```python
from build123d import *

# Parameters (mm, degrees)
BOSS_EXTRUDE1_DEPTH = 3.175
BOSS_EXTRUDE2_DEPTH = 6.35
CAVITY2_START       = -95.885
CAVITY2_OUTLINE_W   = 6.35
CAVITY2_OUTLINE_H   = 6.35
CAVITY2_DEPTH       = 15.875
CAVITY2_START_2     = -64.135
CAVITY2_2_OUTLINE_W = 6.35
CAVITY2_2_OUTLINE_H = 6.35
CAVITY2_2_DEPTH     = 15.875
SKETCH6_R           = 1.3716
CUT_EXTRUDE1_DEPTH  = 175.52022504
SKETCH7_R           = 6.35
CUT_EXTRUDE2_DEPTH  = 175.52022504
SKETCH9_R           = 1.905
CUT_EXTRUDE3_DEPTH  = 175.52022504
SKETCH10_R          = 1.85
CUT_EXTRUDE4_DEPTH  = 175.52022504
CAVITY3_START       = 48.26
CAVITY3_OUTLINE_W   = 6.35
CAVITY3_OUTLINE_H   = 6.35
CAVITY3_DEPTH       = 15.875
CAVITY3_START_2     = 80.01
CAVITY3_2_OUTLINE_W = 6.35
CAVITY3_2_OUTLINE_H = 6.35
CAVITY3_2_DEPTH     = 15.875
CAVITY3_START_3     = -95.885
CAVITY3_3_OUTLINE_W = 6.35
CAVITY3_3_OUTLINE_H = 6.35
CAVITY3_3_DEPTH     = 15.875
CAVITY3_START_4     = -64.135
CAVITY3_4_OUTLINE_W = 6.35
CAVITY3_4_OUTLINE_H = 6.35
CAVITY3_4_DEPTH     = 15.875
CAVITY3_START_5     = -114.3
CAVITY3_5_OUTLINE_W = 6.35
CAVITY3_5_OUTLINE_H = 11.6205
CAVITY3_5_DEPTH     = 2.54
CAVITY3_START_6     = 111.76
CAVITY3_6_OUTLINE_W = 6.35
CAVITY3_6_OUTLINE_H = 11.6205
CAVITY3_6_DEPTH     = 2.54


# Read off the part's stored shape, not the designer's step: Cavity2, Cavity3
with BuildPart() as part:
    # Sketch1 → Boss-Extrude1 (new, symmetric)
    with BuildSketch(Plane(origin=(0, 0, 0), x_dir=(1, 0, 0), z_dir=(0, 1, 0))):
        Polygon((9.874658932, 123.322719821), (-80.219893167, 94.184769753), (-123.322719821, 9.874658932), (-94.184769753, -80.219893167), (-9.874658932, -123.322719821), (80.219893167, -94.184769753), (123.322719821, -9.874658932), (94.184769753, 80.219893167), align=None)
    extrude(amount=BOSS_EXTRUDE1_DEPTH, both=True)

    # Sketch3 → Boss-Extrude2 (add)
    with BuildSketch(Plane(origin=(0, 3.175, 0), x_dir=(1, 0, 0), z_dir=(0, 1, 0))):
        Polygon((95.310120051, 76.74030964), (117.060869008, 83.774833064), (106.89989073, 115.192581558), (57.210976805, 99.122430154), (94.184769753, 80.219893167), align=None)
    extrude(amount=-BOSS_EXTRUDE2_DEPTH)

    # Cavity2 outline → Cavity2 (cut)
    with BuildSketch(Plane(origin=(0, 0, 0), x_dir=(0, 1, 0), z_dir=(0.9514763323416664, 0, -0.3077219345344931)).offset(CAVITY2_START)):
        with Locations((0, 26.416)):
            Rectangle(CAVITY2_OUTLINE_W, CAVITY2_OUTLINE_H)
    extrude(amount=CAVITY2_DEPTH, mode=Mode.SUBTRACT)

    # Cavity2 2 outline → Cavity2 2 (cut)
    with BuildSketch(Plane(origin=(0, 0, 0), x_dir=(0, 1, 0), z_dir=(0.9514763323416664, 0, -0.3077219345344931)).offset(CAVITY2_START_2)):
        with Locations((0, 26.416)):
            Rectangle(CAVITY2_2_OUTLINE_W, CAVITY2_2_OUTLINE_H)
    extrude(amount=CAVITY2_2_DEPTH, mode=Mode.SUBTRACT)

    # Sketch6 → Cut-Extrude1 (cut, through all)
    with BuildSketch(Plane(origin=(0, 3.175, 0), x_dir=(1, 0, 0), z_dir=(0, 1, 0))):
        with Locations(Location((-5.097490915, -79.318746248, 0), (0, 0, 270))):
            Circle(SKETCH6_R)
        with Locations(Location((50.579592916, -61.311929511, 0), (0, 0, 270))):
            Circle(SKETCH6_R)
        with Locations(Location((34.017198322, -10.100999466, 0), (0, 0, 270))):
            Circle(SKETCH6_R)
        with Locations(Location((-21.659885509, -28.107816203, 0), (0, 0, 270))):
            Circle(SKETCH6_R)
    extrude(amount=-CUT_EXTRUDE1_DEPTH, mode=Mode.SUBTRACT)

    # Sketch7 → Cut-Extrude2 (cut, through all)
    with BuildSketch(Plane(origin=(0, 3.175, 0), x_dir=(1, 0, 0), z_dir=(0, 1, 0))):
        with Locations(Location((56.160215938, -31.223340716, 0), (0, 0, 270))):
            Circle(SKETCH7_R)
    extrude(amount=-CUT_EXTRUDE2_DEPTH, mode=Mode.SUBTRACT)

    # Sketch9 → Cut-Extrude3 (cut, through all)
    with BuildSketch(Plane(origin=(0, 3.175, 0), x_dir=(1, 0, 0), z_dir=(0, 1, 0))):
        with Locations(Location((-19.963200574, -76.531714164, 0), (0, 0, 270))):
            Circle(SKETCH9_R)
        with Locations(Location((-41.457577702, -10.07109235, 0), (0, 0, 270))):
            Circle(SKETCH9_R)
        with Locations(Location((60.997920545, -50.347654754, 0), (0, 0, 270))):
            Circle(SKETCH9_R)
        with Locations(Location((39.503543417, 16.11296706, 0), (0, 0, 270))):
            Circle(SKETCH9_R)
    extrude(amount=-CUT_EXTRUDE3_DEPTH, mode=Mode.SUBTRACT)

    # Sketch10 → Cut-Extrude4 (cut, through all)
    with BuildSketch(Plane(origin=(0, 3.175, 0), x_dir=(1, 0, 0), z_dir=(0, 1, 0))):
        with Locations(Location((-1.658619289, 61.997975629, 0), (0, 0, 270))):
            Circle(SKETCH10_R)
        with Locations(Location((-34.960290921, 51.22770792, 0), (0, 0, 270))):
            Circle(SKETCH10_R)
        with Locations(Location((-23.574579343, 16.023083623, 0), (0, 0, 270))):
            Circle(SKETCH10_R)
        with Locations(Location((9.727092289, 26.793351332, 0), (0, 0, 270))):
            Circle(SKETCH10_R)
    extrude(amount=-CUT_EXTRUDE4_DEPTH, mode=Mode.SUBTRACT)

    # Cavity3 outline → Cavity3 (cut)
    with BuildSketch(Plane(origin=(0, 0, 0), x_dir=(0, 1, 0), z_dir=(0.9514763323416664, 0, -0.3077219345344931)).offset(CAVITY3_START)):
        with Locations((0, 26.416)):
            Rectangle(CAVITY3_OUTLINE_W, CAVITY3_OUTLINE_H)
        with Locations((0, -26.416)):
            Rectangle(CAVITY3_OUTLINE_W, CAVITY3_OUTLINE_H)
    extrude(amount=CAVITY3_DEPTH, mode=Mode.SUBTRACT)

    # Cavity3 2 outline → Cavity3 2 (cut)
    with BuildSketch(Plane(origin=(0, 0, 0), x_dir=(0, 1, 0), z_dir=(0.9514763323416664, 0, -0.3077219345344931)).offset(CAVITY3_START_2)):
        with Locations((0, 26.416)):
            Rectangle(CAVITY3_2_OUTLINE_W, CAVITY3_2_OUTLINE_H)
        with Locations((0, -26.416)):
            Rectangle(CAVITY3_2_OUTLINE_W, CAVITY3_2_OUTLINE_H)
    extrude(amount=CAVITY3_2_DEPTH, mode=Mode.SUBTRACT)

    # Cavity3 3 outline → Cavity3 3 (cut)
    with BuildSketch(Plane(origin=(0, 0, 0), x_dir=(0, 1, 0), z_dir=(0.9514763323416664, 0, -0.3077219345344931)).offset(CAVITY3_START_3)):
        with Locations((0, -26.416)):
            Rectangle(CAVITY3_3_OUTLINE_W, CAVITY3_3_OUTLINE_H)
    extrude(amount=CAVITY3_3_DEPTH, mode=Mode.SUBTRACT)

    # Cavity3 4 outline → Cavity3 4 (cut)
    with BuildSketch(Plane(origin=(0, 0, 0), x_dir=(0, 1, 0), z_dir=(0.9514763323416664, 0, -0.3077219345344931)).offset(CAVITY3_START_4)):
        with Locations((0, -26.416)):
            Rectangle(CAVITY3_4_OUTLINE_W, CAVITY3_4_OUTLINE_H)
    extrude(amount=CAVITY3_4_DEPTH, mode=Mode.SUBTRACT)

    # Cavity3 5 outline → Cavity3 5 (cut)
    with BuildSketch(Plane(origin=(0, 0, 0), x_dir=(0, 1, 0), z_dir=(0.9514763323416664, 0, -0.3077219345344931)).offset(CAVITY3_START_5)):
        with Locations((0, 17.43075)):
            Rectangle(CAVITY3_5_OUTLINE_W, CAVITY3_5_OUTLINE_H)
        with Locations((0, -17.43075)):
            Rectangle(CAVITY3_5_OUTLINE_W, CAVITY3_5_OUTLINE_H)
    extrude(amount=CAVITY3_5_DEPTH, mode=Mode.SUBTRACT)

    # Cavity3 6 outline → Cavity3 6 (cut)
    with BuildSketch(Plane(origin=(0, 0, 0), x_dir=(0, 1, 0), z_dir=(0.9514763323416664, 0, -0.3077219345344931)).offset(CAVITY3_START_6)):
        with Locations((0, 17.43075)):
            Rectangle(CAVITY3_6_OUTLINE_W, CAVITY3_6_OUTLINE_H)
        with Locations((0, -17.43075)):
            Rectangle(CAVITY3_6_OUTLINE_W, CAVITY3_6_OUTLINE_H)
    extrude(amount=CAVITY3_6_DEPTH, mode=Mode.SUBTRACT)


solid = part.part
```
Geometry check sheet. Reference: the model listing, model coordinates, mm. A direction names the side the tool comes from. Coordinates: 2 decimals unless noted, no trailing zeros. Order: outer loops, then holes, each group sorted by start corner. A loop starts at its lowest first (then second) coordinate and runs counter-clockwise, first axis right, second up.
Q1. Sectioned sample at C-C on z = -88. Record the cut outline in (x, y) (3 decimals), and give its area (3 significant figures).
Reply:
outline: (-83.382, -3.175) - (115.694, -3.175) - (115.694, 3.175) - (-83.382, 3.175) - close
area: 1,260 mm2
Q2. Thickness scan on probe 1 along Z at (x, y) = (-41, 2.75); probe 2 along X at (y, z) = (0, 27); probe 3 along Z at (x, y) = (-20.5, 0.5). Record the ranges inside material, lowest first.
Reply:
probe 1: z = -106.87 to 8.22, 11.92 to 37.69, 44.36 to 107.41
probe 2: x = -111.4 to -22.47, -20.85 to 51.42, 60.9 to 114.57
probe 3: z = -113.5 to 27.38, 28.84 to 74.7, 78.36 to 117.89
Q3. Tool access check on faces 1 (the face through (-2, 3.175, -2)), 2 (the face through (-46.42, -0.04, 39.44)). Record the directions out of +Z, -Z, +X, -X, +Y, -Y that give a thin tool (end or side, any length) a straight path to the whole face; none if there is none.
Reply:
face 1: +Z, -Z, +X, -X, +Y
face 2: +Y, -Y
Q4. Sectioned sample at A-A on z = 33.5. Record the cut outline in (x, y) (3 decimals).
Reply:
outline: (-109.295, -3.175) - (50.232, -3.175) - (50.232, 3.175) - (-109.295, 3.175) - close; (62.088, -3.175) - (111.244, -3.175) - (111.244, 3.175) - (62.088, 3.175) - close
Q5. Draft check along Z on faces 3 (the face through (83.117, -0.044, -54.598)), 4 (the face through (44.259, -0.044, -45.414)), 5 (the face through (-34.54, 0.04, -108.96)), 6 (the face through (-2, -3.175, -2)). Enter one of: released by +Z, released by -Z, zero draft, split by the parting line, or undercut.
Reply:
face 3: undercut
face 4: undercut
face 5: released by -Z
face 6: zero draft
Q6. Sectioned sample at B-B on y = 1.75. Give the number of separate pieces and of enclosed holes in the cut face, and give its area (3 significant figures).
Reply:
separate pieces: 1
enclosed holes: 21
area: 43,300 mm2
Q7. Depth check by flat-ended pin: pin 1 Ø4.5 at (x, z) = (-41.46, 10.07) entering from +Y (3 decimals); pin 2 Ø3 at (x, y) = (44, 0.5) entering from +Z; pin 3 Ø3 at (x, y) = (-13.5, -1.5) entering from -Z; pin 4 Ø1 at (y, z) = (-1.5, 28) entering from +X. Enter the tip coordinate at first touch or a pass-through.
Reply:
pin 1: stops at y = 3.175
pin 2: stops at z = 106.38
pin 3: stops at z = -116.25
pin 4: stops at x = 114.31
